Can you work these out from the model? Positions are in its coordinate system, mm. A direction names the side the tool comes from. Round coordinates to 2 decimals unless told otherwise and drop trailing zeros. Order: outer loops, then holes, each group sorted by start corner. A loop starts at its lowest first (then second) coordinate and runs counter-clockwise, first axis right, second up. Notation, with made-up numbers: (10.25, 46.5) -> (18.25, 46.5) arc R22 cw to (18.25, 83.5) -> close; hole circle Ø6 at (30.5, 76.5). An arc over 180 degrees is marked (long way). One line per item, written item: value.
```python
from build123d import *

# Parameters (mm, degrees)
SKETCH_1_W          = 200
SKETCH_1_H          = 15
SKETCH_1_R          = 5
EXTRUDE_2_DEPTH     = 40
SKETCH_2_W          = 50
SKETCH_2_H          = 20
CUT_EXTRUDE_2_DEPTH = 40
SKETCH_3_W          = 242.163651579
SKETCH_3_H          = 102.30151502
CUT_EXTRUDE_3_DEPTH = 40


with BuildPart() as part:
    # 草图1 → 凸台-拉伸2 (new body)
    with BuildSketch(Plane.XY):
        with Locations((26.359649123, 8.070175439)):
            Rectangle(SKETCH_1_W, SKETCH_1_H)
        with Locations((-66.300631579, 8.070175439)):
            Circle(SKETCH_1_R, mode=Mode.SUBTRACT)
        with Locations((118.699368421, 8.070175439)):
            Circle(SKETCH_1_R, mode=Mode.SUBTRACT)
    extrude(amount=EXTRUDE_2_DEPTH)

    # 草图2 → 切除-拉伸2 (cut)
    with BuildSketch(Plane(origin=(0, 15.570175439, 0), x_dir=(1, 0, 0), z_dir=(0, 1, 0))):
        with Locations((-73.640350877, -20)):
            Rectangle(SKETCH_2_W, SKETCH_2_H)
        with Locations((126.359649123, -20)):
            Rectangle(SKETCH_2_W, SKETCH_2_H)
    extrude(amount=-CUT_EXTRUDE_2_DEPTH, mode=Mode.SUBTRACT)

    # 草图3 → 切除-拉伸3 (cut)
    with BuildSketch(Plane(origin=(0, 15.570175439, 0), x_dir=(1, 0, 0), z_dir=(0, 1, 0))):
        with Locations((126.359649123, 0)):
            Rectangle(SKETCH_3_W, SKETCH_3_H)
    extrude(amount=-CUT_EXTRUDE_3_DEPTH, mode=Mode.SUBTRACT)

    # 镜向2: part across plane


with BuildPart() as part_1:
    add(part.part)
    add(part.part.mirror(Plane(origin=(5.277823333, -24.429824561, -51.15075751), x_dir=(0, 0, 1), z_dir=(-1, 0, 0))))


solid = part_1.part
```
Q1. Please list where these lines run through material, in increasing order: line 1 along X through (y, z) = (12, 27.5); line 2 along X through (y, z) = (4, 37); line 3 along X through (y, z) = (3.5, 31).
Answers below:
line 1: -48.64 to 59.2
line 2: -73.64 to -69.2, -63.4 to 73.95, 79.76 to 84.2
line 3: -73.64 to -68.33, -64.27 to 74.83, 78.88 to 84.2
Q2. On a 3-axis mill with a long thin cutter (end or side, diameter ignored), from which of +Z, -Z, +X, -X, +Y, -Y can I reach the whole of each face in a straight line? I mean faces 4 (the face through (-59, 8, 30)), 5 (the face through (6, 8, 40)), 6 (the face through (69, 8, 30)). Say none if no direction works.
Answers below:
face 4: -X, +Y, -Y
face 5: +Z, +X, -X, +Y, -Y
face 6: +X, +Y, -Y
Q3. We'd pull the mould along X, two halves only. Please class faces 1 (the face through (69, 8, 10)), 2 (the face through (-61.68, 6.16, 4.93)), 3 (the face through (-48.64, 8, 20)): released by +X, released by -X, zero draft, split by the parting line, or undercut.
Answers below:
face 1: zero draft
face 2: undercut
face 3: released by -X
Q4. I want a section at B-B on y = 4.5. List the corners of the cut face in (x, z) for me, plus the area to 3 significant figures.
Answers below:
outline: (-73.64, 0) -> (-69.8, 0) -> (-69.8, 10) -> (-73.64, 10) -> close; (-73.64, 30) -> (-69.8, 30) -> (-69.8, 40) -> (-73.64, 40) -> close; (-62.8, 0) -> (73.36, 0) -> (73.36, 10) -> (59.2, 10) -> (59.2, 30) -> (73.36, 30) -> (73.36, 40) -> (-62.8, 40) -> (-62.8, 30) -> (-48.64, 30) -> (-48.64, 10) -> (-62.8, 10) -> close; (80.36, 0) -> (84.2, 0) -> (84.2, 10) -> (80.36, 10) -> close; (80.36, 30) -> (84.2, 30) -> (84.2, 40) -> (80.36, 40) -> close
area: 5,030 mm^2
Q5. I want a section at D-D on y = 10.25. List the corners of the cut face in (x, z) for me, plus the area to 3 significant figures.
Answers below:
outline: (-73.64, 0) -> (-70.8, 0) -> (-70.8, 10) -> (-73.64, 10) -> close; (-73.64, 30) -> (-70.8, 30) -> (-70.8, 40) -> (-73.64, 40) -> close; (-61.8, 0) -> (72.36, 0) -> (72.36, 10) -> (59.2, 10) -> (59.2, 30) -> (72.36, 30) -> (72.36, 40) -> (-61.8, 40) -> (-61.8, 30) -> (-48.64, 30) -> (-48.64, 10) -> (-61.8, 10) -> close; (81.36, 0) -> (84.2, 0) -> (84.2, 10) -> (81.36, 10) -> close; (81.36, 30) -> (84.2, 30) -> (84.2, 40) -> (81.36, 40) -> close
area: 4,950 mm^2
Q6. Will these pins go through, and if not, where does the flat tip stop? pin 1 Ø3 at (y, z) = (13.5, 20) entering from -X; pin 2 Ø7.5 at (y, z) = (8.5, 19.5) entering from +X.
Answers below:
pin 1: x = -48.64
pin 2: x = 59.2
Q7. I want a section at A-A on x = -55.5. List the corners of the cut face in (y, z) for me, plus the area to 3 significant figures.
Answers below:
outline: (0.57, 0) -> (15.57, 0) -> (15.57, 10) -> (0.57, 10) -> close; (0.57, 30) -> (15.57, 30) -> (15.57, 40) -> (0.57, 40) -> close
area: 300 mm^2
Q8. I want a section at C-C on z = 34. List the corners of the cut face in (x, y) for me, plus the area to 3 significant figures.
Answers below:
outline: (-73.64, 0.57) -> (84.2, 0.57) -> (84.2, 15.57) -> (-73.64, 15.57) -> close; hole circle Ø10 at (-66.3, 8.07); hole circle Ø10 at (76.86, 8.07)
area: 2,210 mm^2
